from build123d import *

# Parameters (mm, degrees)
SKETCH_1_R           = 13
SKETCH_1_R_2         = 37.5
EXTRUDE_1417_DEPTH   = 16
FILLET_1_R           = 2
FILLET_2_R           = 2
EXTRUDE_2_DEPTH      = 40
EXTRUDE_2_DEPTH_BACK = 56
SKETCH_3_W           = 10
SKETCH_3_H           = 316
CUT_EXTRUDE_1_DEPTH  = 836.425640018
CUT_EXTRUDE_2_DEPTH  = 836.425640018
EXTRUDE_5_DEPTH      = 42
EXTRUDE_5_DEPTH_BACK = 58
EXTRUDE_6_DEPTH      = 14.5
EXTRUDE_6_DEPTH_BACK = 30.5
SKETCH_7_W           = 300
SKETCH_7_H           = 12
SKETCH_8_W           = 150
SKETCH_8_H           = 150
EXTRUDE_7_DEPTH      = 12
EXTRUDE_8_DEPTH      = 16


with BuildPart() as part:
    # 草图1 → Extrude 1417 (new body)
    with BuildSketch(Plane.XY):
        with BuildLine():
            Line((0, -320), (-70, -320))
            ThreePointArc((-70, -320), (-77.071067812, -322.928932188), (-80, -330))
            Line((-80, -330), (-80, -390))
            ThreePointArc((-80, -390), (-77.071067812, -397.071067812), (-70, -400))
            Line((-70, -400), (0, -400))
            Line((0, -400), (0, -720))
            Line((0, -720), (-210, -720))
            Line((-210, -720), (-259.124034735, -327.007722123))
            ThreePointArc((-259.124034735, -327.007722123), (-261.767837242, -322.002574593), (-267.062257748, -320))
            Line((-267.062257748, -320), (-460, -320))
            Line((-460, -320), (-460, 0))
            Line((-460, 0), (-72, 0))
            Line((-72, 0), (-72, -80))
            Line((-72, -80), (0, -80))
            Line((0, -80), (0, -320))
        make_face()
        with Locations((-112, -40)):
            Circle(SKETCH_1_R, mode=Mode.SUBTRACT)
        with Locations((-112, -120)):
            Circle(SKETCH_1_R, mode=Mode.SUBTRACT)
        with Locations((-112, -200)):
            Circle(SKETCH_1_R, mode=Mode.SUBTRACT)
        with Locations((-112, -280)):
            Circle(SKETCH_1_R, mode=Mode.SUBTRACT)
        with Locations((-40, -160)):
            Circle(SKETCH_1_R, mode=Mode.SUBTRACT)
        with Locations((-40, -240)):
            Circle(SKETCH_1_R, mode=Mode.SUBTRACT)
        with Locations((-40, -680)):
            Circle(SKETCH_1_R, mode=Mode.SUBTRACT)
        with Locations((-40, -600)):
            Circle(SKETCH_1_R, mode=Mode.SUBTRACT)
        with Locations((-40, -520)):
            Circle(SKETCH_1_R, mode=Mode.SUBTRACT)
        with Locations((-112, -640)):
            Circle(SKETCH_1_R, mode=Mode.SUBTRACT)
        with Locations((-112, -560)):
            Circle(SKETCH_1_R, mode=Mode.SUBTRACT)
        with Locations((-112, -480)):
            Circle(SKETCH_1_R, mode=Mode.SUBTRACT)
        with Locations((-260, -110)):
            Circle(SKETCH_1_R_2, mode=Mode.SUBTRACT)
    extrude(amount=EXTRUDE_1417_DEPTH)

    # 圆角1
    fillet_1_edges = [part.edges().sort_by_distance(p)[0] for p in [
        (-105, -720, 16),
        (0, -560, 16),
        (-35, -400, 16),
        (-77.071067812, -397.071067812, 16),
        (-80, -360, 16),
        (-77.071067812, -322.928932188, 16),
        (-35, -320, 16),
        (0, -200, 16),
        (-36, -80, 16),
        (-125, -40, 16),
        (-72, -40, 16),
        (-261.767837242, -322.002574593, 16),
        (-266, 0, 16),
        (-125, -120, 16),
        (-460, -160, 16),
        (-125, -200, 16),
        (-363.531128874, -320, 16),
        (-125, -280, 16),
        (-53, -160, 16),
        (-53, -240, 16),
        (-53, -680, 16),
        (-53, -600, 16),
        (-53, -520, 16),
        (-234.562017367, -523.503861062, 16),
        (-125, -640, 16),
        (-125, -560, 16),
        (-125, -480, 16),
        (-297.5, -110, 16),
    ]]
    fillet(fillet_1_edges, radius=FILLET_1_R)

    # 圆角2
    fillet_2_edges = [part.edges().sort_by_distance(p)[0] for p in [
        (-363.531128874, -320, 0),
        (-460, -160, 0),
        (-266, 0, 0),
        (-72, -40, 0),
        (-36, -80, 0),
        (0, -200, 0),
        (-35, -320, 0),
        (-77.071067812, -322.928932188, 0),
        (-80, -360, 0),
        (-77.071067812, -397.071067812, 0),
        (-35, -400, 0),
        (0, -560, 0),
        (-105, -720, 0),
        (-234.562017367, -523.503861062, 0),
        (-261.767837242, -322.002574593, 0),
        (-125, -40, 0),
        (-125, -120, 0),
        (-125, -200, 0),
        (-125, -280, 0),
        (-53, -160, 0),
        (-53, -240, 0),
        (-53, -680, 0),
        (-53, -600, 0),
        (-53, -520, 0),
        (-125, -640, 0),
        (-125, -560, 0),
        (-125, -480, 0),
        (-297.5, -110, 0),
    ]]
    fillet(fillet_2_edges, radius=FILLET_2_R)

    # 草图3 → 凸台-拉伸2 (add, two sides: drawn at the far end of the back side and taken through both)
    with BuildSketch(Plane.XY.offset(16).offset(-EXTRUDE_2_DEPTH_BACK)):
        with Locations((-415, -160)):
            Rectangle(SKETCH_3_W, SKETCH_3_H)
        with Locations((-365, -160)):
            Rectangle(SKETCH_3_W, SKETCH_3_H)
    extrude(amount=EXTRUDE_2_DEPTH + EXTRUDE_2_DEPTH_BACK)

    # 草图4 → 切除-拉伸1 (cut, through all)
    with BuildSketch(Plane.ZY.offset(420)):
        Polygon((-20, -2), (-45.5, -32), (-45.5, -2), align=None)
    extrude(amount=-CUT_EXTRUDE_1_DEPTH, mode=Mode.SUBTRACT)

    # 草图5 → 切除-拉伸2 (cut, through all)
    with BuildSketch(Plane.ZY.offset(420)):
        Polygon((36, -2), (56, -32), (56, -2), align=None)
    extrude(amount=-CUT_EXTRUDE_2_DEPTH, mode=Mode.SUBTRACT)

    # 草图6 → 凸台-拉伸5 (add, two sides: drawn at the far end of the back side and taken through both)
    with BuildSketch(Plane.XY.offset(16).offset(-EXTRUDE_5_DEPTH_BACK)):
        Polygon((-267.062257748, -318), (-460, -318), (-460, -330), (-277.426505546, -330), (-220.363518026, -718), (-208.234435563, -718), align=None)
    extrude(amount=EXTRUDE_5_DEPTH + EXTRUDE_5_DEPTH_BACK)

    # 草图7 → 凸台-拉伸6 (add, two sides: drawn at the far end of the back side and taken through both)
    with BuildSketch(Plane(origin=(0, 0, 0), x_dir=(-1, 0, 0), z_dir=(0, 0, -1)).offset(-EXTRUDE_6_DEPTH_BACK)):
        with Locations((308, 4)):
            Rectangle(SKETCH_7_W, SKETCH_7_H)
    extrude(amount=EXTRUDE_6_DEPTH + EXTRUDE_6_DEPTH_BACK)

    # 草图8 → 凸台-拉伸7 (add)
    with BuildSketch(Plane.XZ.offset(330)):
        with Locations((-385, 8)):
            Rectangle(SKETCH_8_W, SKETCH_8_H)
    extrude(amount=EXTRUDE_7_DEPTH)

    # 草图9 → 凸台-拉伸8 (add)
    with BuildSketch(Plane.XY.offset(16)):
        Polygon((0, -720), (0, -400), (-70, -400), (-80, -390), (-80, -330), (-70, -320), (0, -320), (0, -80), (-72, -80), (-72, 0), (-360, -2), (-360, -318), (-267.062257748, -318), (-207.940296452, -720), align=None)
    extrude(amount=-EXTRUDE_8_DEPTH)


solid = part.part
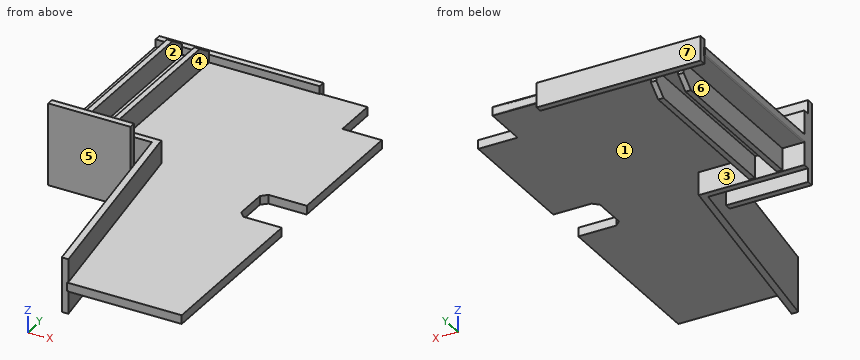
For this review, take the finished solid that the model builds, in its own axes (mm). Face numbers are marked on the shaded views. A direction names the side the tool comes from. Round coordinates to 2 decimals unless told otherwise and drop trailing zeros. Order: outer loops, then holes, each group sorted by start corner. A loop starts at its lowest first (then second) coordinate and runs counter-clockwise, first axis right, second up. Notation, with made-up numbers: (26.25, 36) -> (66.25, 36) arc R20 ccw to (66.25, 60) -> close; hole circle Ø8 at (83.5, -19). An arc over 180 degrees is marked (long way). Write item = value, one per line. Start each with the question number.
1) Take a section at A-A on x = -36.5. State the section outline as (y, z) points, plus the area to 3 significant figures.
2) Take a section at B-B on y = -236. State the section outline as (x, z) points, plus the area to 3 significant figures.
3) Insertion check: pin 1 (1.6 mm diameter, centred on x = -459.5, z = 8.5, fed in from +Y); pin 2 (1.5 mm diameter, centred on x = -228, y = -462.5, fed in from -Z); pin 3 (1.5 mm diameter, centred on y = -406, z = -4, fed in from +X). Each pin has a flat end and moves straight along its axis. Give the tip position at first contact, or say it passes through.
4) Tool access review of the marked faces 5, 6 and 7: name each direction out of +Z, -Z, +X, -X, +Y, -Y from which nothing blocks a thin tool from reaching the whole face with its end or side.
5) To check wall thickness, follow line 1 (X direction, y = -193, z = -38); line 2 (Y direction, x = -22.5, z = 9); line 3 (Y direction, x = -383, z = -46). State the ranges of each line that lie inside material, in increasing order. Write a range as from..to.
6) The part is to be moulded in two halves that separate along X. For the marked faces 1, 2, 3 and 4, say which applies: +X half, -X half, draft (parallel to the pull), parting line (faces both ways), or undercut.
7) Take a section at D-D on y = -542. State the section outline as (x, z) points.
8) Take a section at C-C on x = -340. State the section outline as (y, z) points.
Verdict:
q1.outline = (-720, 0) -> (-400, 0) -> (-400, 16) -> (-720, 16) -> close; (-320, 0) -> (-80, 0) -> (-80, 16) -> (-320, 16) -> close
q1.area = 8,960 mm2
q2.outline = (-460, 2) arc R2 ccw to (-458, 0) -> (-420, 0) -> (-420, -40) -> (-410, -40) -> (-410, 0) -> (-370, 0) -> (-370, -40) -> (-360, -40) -> (-360, 0) -> (0, 0) -> (0, 16) -> (-360, 16) -> (-360, 56) -> (-370, 56) -> (-370, 16) -> (-410, 16) -> (-410, 56) -> (-420, 56) -> (-420, 16) -> (-458, 16) arc R2 ccw to (-460, 14) -> close
q2.area = 8,960 mm2
q3.pin_1 = 0
q3.pin_2 = 0
q3.pin_3 = -254.01
q4.face_5 = +Z, -Z, -X, -Y
q4.face_6 = -Z, -X
q4.face_7 = +Z, -Z, +X, -X, +Y
q5.line_1 = -420..-410, -370..-360
q5.line_2 = -720..-400, -320..-80
q5.line_3 = -342..-330
q6.face_1 = draft
q6.face_2 = undercut
q6.face_3 = undercut
q6.face_4 = +X half
q7.outline = (-246.25, -42) -> (-234.12, -42) -> (-234.12, 0) -> (0, 0) -> (0, 16) -> (-234.12, 16) -> (-234.12, 58) -> (-246.25, 58) -> close
q8.outline = (-342, -67) -> (-330, -67) -> (-330, -42) -> (-318, -42) -> (-318, 0) -> (-2, 0) -> (-2, -14.5) -> (10, -14.5) -> (10, 30.5) -> (-2, 30.5) -> (-2, 16) -> (-318, 16) -> (-318, 58) -> (-330, 58) -> (-330, 83) -> (-342, 83) -> close
